Autodesk Inventor part; units mm, degrees
ref_plane "YZ Plane" through (0, 0, 0) normal (1, 0, 0) x (0, 1, 0)
ref_plane "XZ Plane" through (0, 0, 0) normal (0, 1, 0) x (-1, 0, 0)
ref_plane "XY Plane" through (0, 0, 0) normal (0, 0, 1) x (1, 0, 0)
sketch "Sketch1" plane through (0, 0, 0) normal (0, 0, 1) x (1, 0, 0)
  line L0 (0.4379, 0) -> (32.5379, 0)
  line L1 (32.5379, 0) -> (32.5379, 14.1)
  line L2 (32.5379, 14.1) -> (0.4379, 14.1)
  line L3 (0.4379, 14.1) -> (0.4379, 0)
  circle A0 centre (7.5379, 7.05) radius 1.5
  point P0 (0, 0)
  dimension "d0" = 14.1
  dimension "d2" = 32.1
  dimension "d3" = 3
  dimension "d4" = 7.1
  dimension "d5" = 7.05
extrude "Extrusion1" add sketch "Sketch1" along normal blind 1.6
sketch "Sketch2" plane through (0, 0, 1.6) normal (0, 0, 1) x (1, 0, 0)
  line L0 (0.4379, 0) -> (32.5379, 0)
  line L1 (26.5379, 0) -> (32.5379, 0)
  line L2 (32.5379, 0) -> (32.5379, 14.1)
  line L3 (32.5379, 14.1) -> (26.5379, 14.1)
  line L4 (26.5379, 14.1) -> (26.5379, 0)
  point P0 (0, 0)
  dimension "d8" = 6
extrude "Extrusion2" add sketch "Sketch2" along normal blind 2
sketch "Sketch3" plane through (0, 0, 3.6) normal (0, 0, 1) x (1, 0, 0)
  line L0 (26.5379, 0) -> (32.5379, 0)
  line L1 (32.5379, 0) -> (32.5379, 14.1)
  line L2 (26.5379, 14.1) -> (32.5379, 14.1)
  line L3 (32.5379, 14.1) -> (32.5379, 10.1)
  line L4 (32.5379, 10.1) -> (26.5379, 10.1)
  line L5 (26.5379, 10.1) -> (26.5379, 14.1)
  line L6 (26.5379, 0) -> (32.5379, 0)
  line L7 (32.5379, 0) -> (32.5379, 4)
  line L8 (32.5379, 4) -> (26.5379, 4)
  line L9 (26.5379, 4) -> (26.5379, 0)
  point P0 (0, 0)
  dimension "d12" = 4
  dimension "d14" = 4
extrude "Extrusion3" add sketch "Sketch3" along normal blind 8.2
properties part number "optical sensor pcb"
Could you check a few things on this model? Use its own coordinates, in mm. A direction names the side the tool comes from. Give positions to 0.01 mm unless a question says otherwise; leave off trailing zeros. Write each loop counter-clockwise with the first axis right and the second up, starting at its lowest first coordinate (ties: lowest second). Pieces come first, ordered by that corner, then holes. Notation, with made-up numbers: (-11, 19.25) - (39, 19.25) arc R28 ccw to (39, 57.25) - close; hole circle Ø11 at (65, -5.5). An arc over 180 degrees is marked (long way). Use CSV: the item, a comma, the result in double quotes. Start each with the question number.
Item 1: I'm going to push flat-ended pins straight in: pin 1 (3 mm diameter, centred on x = 30.5, y = 7.5, fed in from +Z); pin 2 (5 mm diameter, centred on x = 7.54, y = 7.05, fed in from +Z); pin 3 (4 mm diameter, centred on y = 12.5, z = 8, fed in from -X). Where does each tip first touch, or does it pass through?
Item 2: If we mould it in two halves opening along Y, with no side actions, what happens to faces 4 (the face through (29, 7, 3.6)), 5 (the face through (8.924, 7.625, 0.789)), 6 (the face through (24, 14.1, 1)), 7 (the face through (16, 7, 0))? For each: pulls with the +Y half, pulls with the -Y half, needs draft (parallel to the pull), parting line crosses it, or undercut.
Item 3: I want a section at D-D, the plane y = 11.5. Please give me the cut outline in (x, z).
Item 4: I want a section at C-C, the plane x = 8.5. Please give me the cut outline in (y, z).
Item 5: I want a section at B-B, the plane y = 7.05. Please give me the cut outline in (x, z), then the cut area to 3 significant figures.
Item 6: For faces 1 (the face through (32.538, 7, 3)), 2 (the face through (26.538, 10.3, 5.5)), 3 (the face through (30, 4, 8)), which set-ups out of +Z, -Z, +X, -X, +Y, -Y let a thin tool reach every point of the face, with its end or its side?
Item 7: If I drill on line 1 along Y through (x, z) = (31, 10); line 2 along Z through (x, y) = (20, 3); line 3 along X through (y, z) = (1.5, 5.75), over which ranges is the centre line in solid material (lowest first)?
Item 8: I want a section at A-A, the plane z = 8.5. Please give me the cut outline in (x, y), then the cut area to 3 significant figures.
Findings:
1,pin 1,"stops at z = 3.6"
1,pin 2,"stops at z = 1.6"
1,pin 3,"stops at x = 26.54"
2,face 4,"undercut"
2,face 5,"undercut"
2,face 6,"pulls with the +Y half"
2,face 7,"needs draft"
3,outline,"(0.44, 0) - (32.54, 0) - (32.54, 11.8) - (26.54, 11.8) - (26.54, 1.6) - (0.44, 1.6) - close"
4,outline,"(0, 0) - (5.9, 0) - (5.9, 1.6) - (0, 1.6) - close; (8.2, 0) - (14.1, 0) - (14.1, 1.6) - (8.2, 1.6) - close"
5,outline,"(0.44, 0) - (6.04, 0) - (6.04, 1.6) - (0.44, 1.6) - close; (9.04, 0) - (32.54, 0) - (32.54, 3.6) - (26.54, 3.6) - (26.54, 1.6) - (9.04, 1.6) - close"
5,area,"58.6 mm2"
6,face 1,"+Z, -Z, +X, +Y, -Y"
6,face 2,"+Z, -X, +Y, -Y"
6,face 3,"+Z, +X, -X"
7,line 1,"y = 0 to 4, 10.1 to 14.1"
7,line 2,"z = 0 to 1.6"
7,line 3,"x = 26.54 to 32.54"
8,outline,"(26.54, 0) - (32.54, 0) - (32.54, 4) - (26.54, 4) - close; (26.54, 10.1) - (32.54, 10.1) - (32.54, 14.1) - (26.54, 14.1) - close"
8,area,"48.0 mm2"
